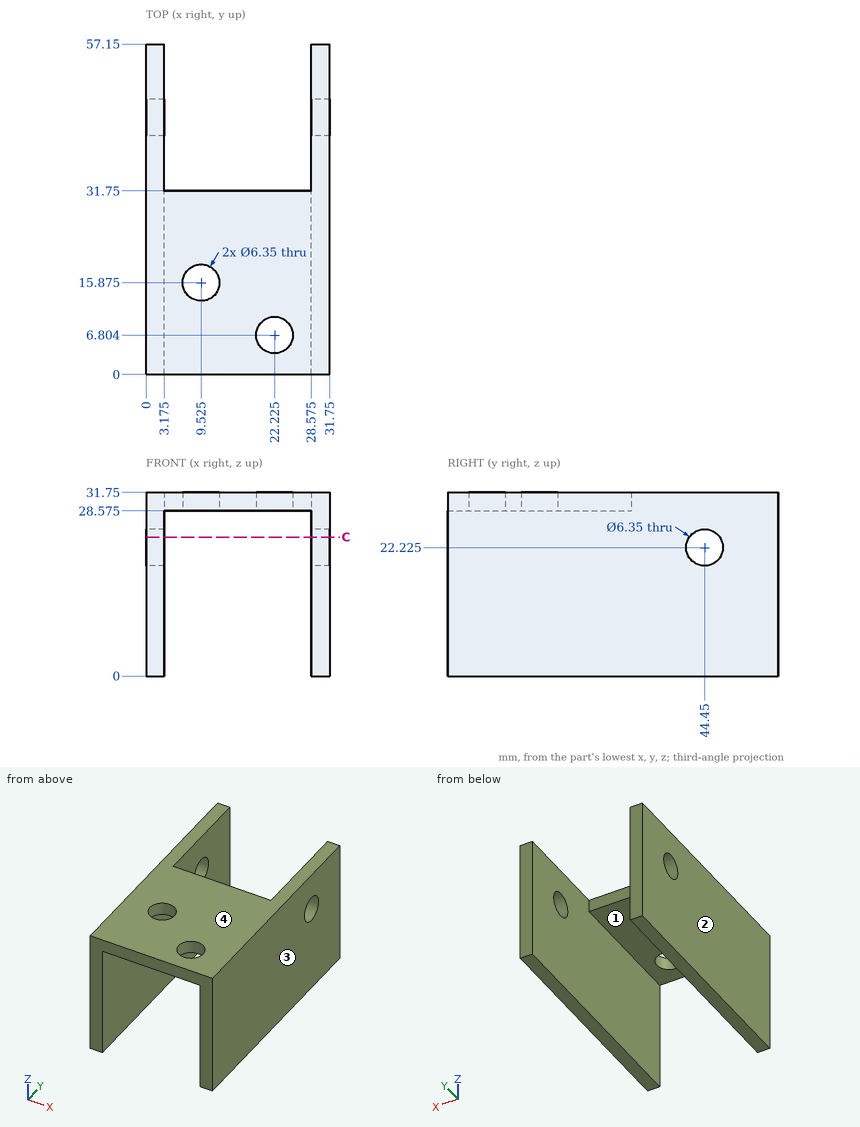
Could you check a few things on this drawing? It's one solid part, dimensions in mm from its lowest x, y, z. Coordinates: 2 decimals unless noted, no trailing zeros.
1) I'm going to push flat-ended pins straight in: pin 1 (5.5 mm diameter, centred on x = 22.22, y = 6.8, fed in from -Z); pin 2 (8.5 mm diameter, centred on x = 9.525, y = 15.875, fed in from -Z) (3 decimals); pin 3 (3.5 mm diameter, centred on x = 18, z = 31, fed in from +Y). Where does each tip first touch, or does it pass through?
Filled in:
pin 1: passes through
pin 2: stops at z = 28.575
pin 3: stops at y = 31.75
2) If I drill on line 1 (Z direction, x = 30, y = 44); line 2 (X direction, y = 6, z = 30); line 3 (Y direction, x = 30, z = 23.5), over which ranges is the centre line in solid material (lowest first)?
Filled in:
line 1: z = 0 to 19.08, 25.37 to 31.75
line 2: x = 0 to 19.15, 25.3 to 31.75
line 3: y = 0 to 41.54, 47.36 to 57.15
3) Thinking about a two-plate mould opening in X: for the marked faces 1, 2, 3 and 4, which applies, +X half, -X half, draft (parallel to the pull), parting line (faces both ways), or undercut?
Filled in:
face 1: undercut
face 2: -X half
face 3: +X half
face 4: draft
4) If we section it at C-C (z = 24): Count the separate pieces of the cut face and the enclosed holes in it.
Filled in:
separate pieces: 4
enclosed holes: 0
